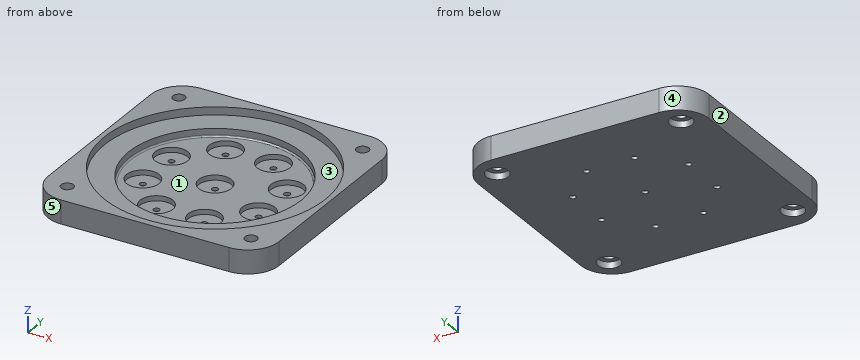
from build123d import *

# Parameters (mm, degrees)
BOSS_EXTRUDE1_DEPTH                     = 19.05
INSET_START                             = 19.05
SKETCH4_R                               = 89.662
INSET_RIM_DEPTH                         = 6.35
CUT_EXTRUDE1_START                      = 12.7
SKETCH9_R                               = 69.85
CUT_EXTRUDE1_DEPTH                      = 6.35
FILLET2_R                               = 1.27
CBORE_FOR_M8_HEX_HEAD_BOLT1_D           = 10
CBORE_FOR_M8_HEX_HEAD_BOLT1_CBORE_D     = 18.011
CBORE_FOR_M8_HEX_HEAD_BOLT1_CBORE_DEPTH = 5.3
SKETCH12_R                              = 2.54
CUT_EXTRUDE2_DEPTH                      = 6.35
SKETCH13_R                              = 13.208
SKETCH13_R_2                            = 2.54
CUT_EXTRUDE3_DEPTH                      = 4.064


with BuildPart() as part:
    # Sketch1 → Boss-Extrude1 (new body)
    with BuildSketch(Plane.XY):
        with BuildLine():
            Line((93.6625, 69.85), (93.6625, -69.85))
            ThreePointArc((93.6625, -69.85), (86.223012242, -87.810512242), (68.2625, -95.25))
            Line((68.2625, -95.25), (-68.2625, -95.25))
            ThreePointArc((-68.2625, -95.25), (-86.223012242, -87.810512242), (-93.6625, -69.85))
            Line((-93.6625, -69.85), (-93.6625, 69.85))
            ThreePointArc((-93.6625, 69.85), (-86.223012242, 87.810512242), (-68.2625, 95.25))
            Line((-68.2625, 95.25), (68.2625, 95.25))
            ThreePointArc((68.2625, 95.25), (86.223012242, 87.810512242), (93.6625, 69.85))
        make_face()
    extrude(amount=BOSS_EXTRUDE1_DEPTH)

    # Sketch4 → Inset Rim (cut)
    with BuildSketch(Plane.XY.offset(INSET_START)):
        Circle(SKETCH4_R)
    extrude(amount=-INSET_RIM_DEPTH, mode=Mode.SUBTRACT)

    # Sketch9 → Cut-Extrude1 (cut)
    with BuildSketch(Plane.XY.offset(CUT_EXTRUDE1_START)):
        Circle(SKETCH9_R)
    extrude(amount=-CUT_EXTRUDE1_DEPTH, mode=Mode.SUBTRACT)

    # Fillet2
    fillet2_edges = [part.edges().sort_by_distance(p)[0] for p in [
        (-69.85, 0, 6.35),
    ]]
    fillet(fillet2_edges, radius=FILLET2_R)

    # CBORE for M8 Hex Head Bolt1 (through all)
    with Locations(Plane(origin=(0, 0, 0), x_dir=(-1, 0, 0), z_dir=(0, 0, -1))):
        with Locations((-74.521339476, -75.893393448), (-74.521339476, 75.893393448), (74.521339476, 75.893393448), (74.521339476, -75.893393448)):
            CounterBoreHole(CBORE_FOR_M8_HEX_HEAD_BOLT1_D / 2, CBORE_FOR_M8_HEX_HEAD_BOLT1_CBORE_D / 2, CBORE_FOR_M8_HEX_HEAD_BOLT1_CBORE_DEPTH)

    # Sketch12 → Cut-Extrude2 (cut)
    with BuildSketch(Plane(origin=(0, 0, 0), x_dir=(-1, 0, 0), z_dir=(0, 0, -1))):
        Circle(SKETCH12_R)
        with Locations((19.440318364, 46.933080252)):
            Circle(SKETCH12_R)
        with Locations((46.933080827, 19.440319753)):
            Circle(SKETCH12_R)
        with Locations((46.933082215, -19.440316401)):
            Circle(SKETCH12_R)
        with Locations((19.440321716, -46.933078863)):
            Circle(SKETCH12_R)
        with Locations((-19.440314437, -46.933080252)):
            Circle(SKETCH12_R)
        with Locations((-46.9330769, -19.440319753)):
            Circle(SKETCH12_R)
        with Locations((-46.933078288, 19.440316401)):
            Circle(SKETCH12_R)
        with Locations((-19.440317789, 46.933078863)):
            Circle(SKETCH12_R)
    extrude(amount=-CUT_EXTRUDE2_DEPTH, mode=Mode.SUBTRACT)

    # Sketch13 → Cut-Extrude3 (cut)
    with BuildSketch(Plane.XY.offset(6.35)):
        with Locations((46.933078863, 19.440317789)):
            Circle(SKETCH13_R)
        with Locations((46.933078288, 19.440316401)):
            Circle(SKETCH13_R_2, mode=Mode.SUBTRACT)
        with Locations((19.440317789, 46.933078863)):
            Circle(SKETCH13_R)
        with Locations((19.440317789, 46.933078863)):
            Circle(SKETCH13_R_2, mode=Mode.SUBTRACT)
        with Locations((46.933078863, -19.440317789)):
            Circle(SKETCH13_R)
        with Locations((46.9330769, -19.440319753)):
            Circle(SKETCH13_R_2, mode=Mode.SUBTRACT)
        with Locations((19.440317789, -46.933078863)):
            Circle(SKETCH13_R)
        with Locations((19.440314437, -46.933080252)):
            Circle(SKETCH13_R_2, mode=Mode.SUBTRACT)
        Circle(SKETCH13_R)
        Circle(SKETCH13_R_2, mode=Mode.SUBTRACT)
        with Locations((-19.440317789, -46.933078863)):
            Circle(SKETCH13_R)
        with Locations((-19.440321716, -46.933078863)):
            Circle(SKETCH13_R_2, mode=Mode.SUBTRACT)
        with Locations((-46.933078863, -19.440317789)):
            Circle(SKETCH13_R)
        with Locations((-46.933082215, -19.440316401)):
            Circle(SKETCH13_R_2, mode=Mode.SUBTRACT)
        with Locations((-46.933078863, 19.440317789)):
            Circle(SKETCH13_R)
        with Locations((-46.933080827, 19.440319753)):
            Circle(SKETCH13_R_2, mode=Mode.SUBTRACT)
        with Locations((-19.440317789, 46.933078863)):
            Circle(SKETCH13_R)
        with Locations((-19.440318364, 46.933080252)):
            Circle(SKETCH13_R_2, mode=Mode.SUBTRACT)
    extrude(amount=-CUT_EXTRUDE3_DEPTH, mode=Mode.SUBTRACT)


solid = part.part
Geometry check sheet. Reference: the model listing, model coordinates, mm. Face numbers are marked on the shaded views. A direction names the side the tool comes from. Coordinates: 2 decimals unless noted, no trailing zeros. Order: outer loops, then holes, each group sorted by start corner. A loop starts at its lowest first (then second) coordinate and runs counter-clockwise, first axis right, second up. Notation, with made-up numbers: (27.5, 37.5) - (70.5, 37.5) arc R25 ccw to (70.5, 60.5) - close; hole circle Ø10 at (82, 38). An arc over 180 degrees is marked (long way). Answer in a Markdown table with one row per item. Add a question column.
1) Gauge pin test, flat ends, axial feed: P1, Ø8, axis at x = 4, y = -6, coming from the +Z side; P2, Ø5.5, axis at x = 72.5, y = -78.5, coming from the -Z side; P3, Ø1.5, axis at x = 74.5, z = 6, coming from the +Y side. Record the tip position at first contact, or that the pin passes through.
2) Release check for a two-part mould opening along Y. For the marked faces 3, 4 and 5 record: +Y half, -Y half, draft (parallel to the pull), parting line (faces both ways), or undercut.
3) Cross-section at B-B, the plane x = 0. Record the cut outline in (y, z).
4) Cross-section at C-C, the plane z = 10.5. Record the cut outline in (x, y).
5) Material ranges on line 1 along Y through (x, z) = (19, 2.5); line 2 along X through (y, z) = (30, 5.5); line 3 along X through (y, z) = (-30.5, 2.5), recorded low to high. Write a range as [from, to].
6) Cross-section at A-A, the plane y = 0. Record the cut outline in (x, z), then the cut area to 3 significant figures.
7) Set-up check for the marked faces 1 and 2: record each of +Z, -Z, +X, -X, +Y, -Y from which the full face is reachable in a straight line by a thin tool's end or side.
Check result:
| question | item | result |
|---|---|---|
| 1 | P1 | stops at z = 2.29 |
| 1 | P2 | stops at z = 5.3 |
| 1 | P3 | stops at y = 94.65 |
| 2 | face 3 | undercut |
| 2 | face 4 | +Y half |
| 2 | face 5 | -Y half |
| 3 | outline | (-95.25, 0) - (-2.54, 0) - (-2.54, 2.29) - (-13.21, 2.29) - (-13.21, 6.35) - (-68.58, 6.35) arc R1.27 cw to (-69.85, 7.62) - (-69.85, 12.7) - (-89.66, 12.7) - (-89.66, 19.05) - (-95.25, 19.05) - close; (2.54, 0) - (95.25, 0) - (95.25, 19.05) - (89.66, 19.05) - (89.66, 12.7) - (69.85, 12.7) - (69.85, 7.62) arc R1.27 cw to (68.58, 6.35) - (13.21, 6.35) - (13.21, 2.29) - (2.54, 2.29) - close |
| 4 | outline | (-93.66, -69.85) arc R25.4 ccw to (-68.26, -95.25) - (68.26, -95.25) arc R25.4 ccw to (93.66, -69.85) - (93.66, 69.85) arc R25.4 ccw to (68.26, 95.25) - (-68.26, 95.25) arc R25.4 ccw to (-93.66, 69.85) - close; hole circle Ø10 at (-74.52, -75.89); hole circle Ø10 at (-74.52, 75.89); hole circle Ø139.7 at (0, 0); hole circle Ø10 at (74.52, -75.89); hole circle Ø10 at (74.52, 75.89) |
| 5 | line 1 | y = [-95.25, -60.13], [-33.73, 33.73], [60.13, 95.25] |
| 5 | line 2 | x = [-93.66, -54.87], [-39, 39], [54.87, 93.66] |
| 5 | line 3 | x = [-93.66, -54.15], [-39.71, 39.71], [54.15, 93.66] |
| 6 | outline | (-93.66, 0) - (-2.54, 0) - (-2.54, 2.29) - (-13.21, 2.29) - (-13.21, 6.35) - (-68.58, 6.35) arc R1.27 cw to (-69.85, 7.62) - (-69.85, 12.7) - (-89.66, 12.7) - (-89.66, 19.05) - (-93.66, 19.05) - close; (2.54, 0) - (93.66, 0) - (93.66, 19.05) - (89.66, 19.05) - (89.66, 12.7) - (69.85, 12.7) - (69.85, 7.62) arc R1.27 cw to (68.58, 6.35) - (13.21, 6.35) - (13.21, 2.29) - (2.54, 2.29) - close |
| 6 | area | 1,420 mm² |
| 7 | face 1 | +Z |
| 7 | face 2 | +Z, -Z, -X, +Y, -Y |
